Check sheet for the modelled part. Datum: model origin and axes. Units: mm. Round coordinates to 2 decimals unless told otherwise and drop trailing zeros. Write each loop counter-clockwise with the first axis right and the second up, starting at its lowest first coordinate (ties: lowest second). Pieces come first, ordered by that corner, then holes.
Item 1: Cross-section at C-C on z = -0.25. Enter the section's corners in (x, y), plus the area to 3 significant figures.
Item 2: Go/stop test with flat-tipped pins: pin 1 Ø0.5 at (y, z) = (-12, 0) entering from +X; pin 2 Ø1.6 at (x, y) = (-4.25, -11.03) entering from +Z. Record where each tip stops, or that it passes through.
Item 3: Cross-section at D-D on y = -0.67. Enter the section's corners in (x, z), plus the area to 3 significant figures.
Item 4: Cross-section at B-B on y = 4.5. Enter the section's corners in (x, z).
Item 5: Cross-section at A-A on x = -4.25. Enter the section's corners in (y, z).
Item 6: Material ranges on line 1 (X direction, y = -11, z = 0.25); line 2 (Y direction, x = 4.25, z = -0.2); line 3 (Y direction, x = 0, z = -0.1), recorded low to high.
from build123d import *

# Parameters (mm, degrees)
EXTRUDE_991_DEPTH      = 0.5
EXTRUDE_991_DEPTH_BACK = 0.5
SKETCH_1_R             = 1


with BuildPart() as part:
    # Sketch 1 → Extrude 991 (new, two sides: drawn at the far end of the back side and taken through both)
    with BuildSketch(Plane.XY.offset(-EXTRUDE_991_DEPTH_BACK)):
        with BuildLine():
            Line((-1.25, -9.83515139), (-1.25, -14.315530029))
            ThreePointArc((-1.25, -14.315530029), (-4.355811387, -13.693933225), (-7.25, -12.407030265))
            ThreePointArc((-7.25, -12.407030265), (-7.042959472, -9.929441632), (-8.18310536, -7.720057427))
            ThreePointArc((-8.18310536, -7.720057427), (0, 11.25), (8.18310536, -7.720057427))
            ThreePointArc((8.18310536, -7.720057427), (7.042959472, -9.929441632), (7.25, -12.407030265))
            ThreePointArc((7.25, -12.407030265), (4.355811387, -13.693933225), (1.25, -14.315530029))
            Line((1.25, -14.315530029), (1.25, -9.83515139))
            ThreePointArc((1.25, -9.83515139), (0, 8.58), (-1.25, -9.83515139))
        make_face()
        with Locations((-4.25, -11.032311518)):
            Circle(SKETCH_1_R, mode=Mode.SUBTRACT)
        with Locations(Location((4.25, -11.032311518, 0), (0, 0, 180))):
            Circle(SKETCH_1_R, mode=Mode.SUBTRACT)
    extrude(amount=EXTRUDE_991_DEPTH + EXTRUDE_991_DEPTH_BACK)


solid = part.part
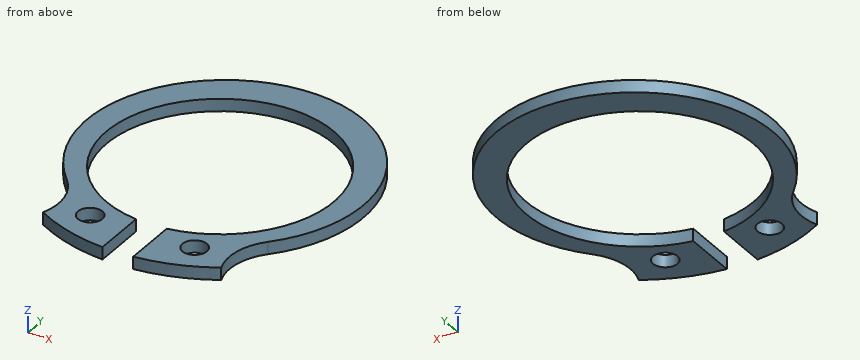
Response values:
1. outline: (-8.18, -7.72) arc R4.5 cw to (-7.25, -12.41) arc R14.37 ccw to (-1.25, -14.32) - (-1.25, -9.84) arc R9.25 cw (long way) to (1.25, -9.84) - (1.25, -14.32) arc R14.37 ccw to (7.25, -12.41) arc R4.5 cw to (8.18, -7.72) arc R11.25 ccw (long way) to start; hole circle Ø2 at (-4.25, -11.03); hole circle Ø2 at (4.25, -11.03)
1. area: 159 mm2
2. pin 1: stops at x = 7.19
2. pin 2: passes through
3. outline: (-11.23, -0.5) - (-9.25, -0.5) - (-9.25, 0.5) - (-11.23, 0.5) - close; (9.25, -0.5) - (11.23, -0.5) - (11.23, 0.5) - (9.25, 0.5) - close
3. area: 3.96 mm2
4. outline: (-10.31, -0.5) - (-7.67, -0.5) - (-7.67, 0.5) - (-10.31, 0.5) - close; (7.67, -0.5) - (10.31, -0.5) - (10.31, 0.5) - (7.67, 0.5) - close
5. outline: (-13.73, -0.5) - (-12.03, -0.5) - (-12.03, 0.5) - (-13.73, 0.5) - close; (-10.03, -0.5) - (-8.89, -0.5) - (-8.89, 0.5) - (-10.03, 0.5) - close; (7.55, -0.5) - (10.42, -0.5) - (10.42, 0.5) - (7.55, 0.5) - close
6. line 1: x = -6.96 to -5.25, -3.25 to -1.25, 1.25 to 3.25, 5.25 to 6.96
6. line 2: y = -13.73 to -12.03, -10.03 to -8.89, 7.55 to 10.42
6. line 3: y = 8.58 to 11.25
